CAD build for the part. Positions are in the model's coordinates, mm. Face numbers are marked on the shaded views. Coordinates: 2 decimals unless noted, no trailing zeros. Order: outer loops, then holes, each group sorted by start corner. A loop starts at its lowest first (then second) coordinate and runs counter-clockwise, first axis right, second up. Notation, with made-up numbers: M -4.75,60 L 13.25,60 A5 cw 13.25,64 Z; hole C -35.75,42.25 d3. An arc over 180 degrees is marked long. Write item = value, one per line.
from build123d import *

# Parameters (mm, degrees)
F1_R      = 645.16
F3_DEPTH  = 64.516
F2_R      = 241.935
F4_DEPTH  = 645.16
F0_R      = 65.151
F5_DEPTH  = 645.161
F6_R      = 64.516377
F7_DEPTH  = 127000
F8_R      = 32.258
F10_DEPTH = 64.516
F9_R      = 32.893
F11_DEPTH = 65.786


with BuildPart() as f3:
    # F1 (on Top) → F3 (new body)
    with BuildSketch(Plane.XY):
        Circle(F1_R)
    extrude(amount=F3_DEPTH)

    # F2 (on Top) → F4 (join)
    with BuildSketch(Plane.XY):
        Circle(F2_R)
    extrude(amount=F4_DEPTH)

    # F0 (on Top) → F5 (cut, through all)
    with BuildSketch(Plane.XY):
        Circle(F0_R)
    extrude(amount=F5_DEPTH, mode=Mode.SUBTRACT)

    # F6 (on Right) → F7 (cut, symmetric)
    with BuildSketch(Plane.YZ):
        with Locations((0, 322.58)):
            Circle(F6_R)
    extrude(amount=F7_DEPTH, both=True, mode=Mode.SUBTRACT)

    # F8 (on face) → F10 (join)
    with BuildSketch(Plane.XY.offset(645.16)):
        with Locations((0, 161.29)):
            Circle(F8_R)
    extrude(amount=F10_DEPTH)

    # F9 (on face) → F11 (cut)
    with BuildSketch(Plane.XY.offset(645.16)):
        with Locations((0, -161.29)):
            Circle(F9_R)
    extrude(amount=-F11_DEPTH, mode=Mode.SUBTRACT)


with BuildPart() as f12_1:
    # F12: copy of F3
    add(f3.part.moved(Location((1879.6, 0, 0))))


solid = f3.part
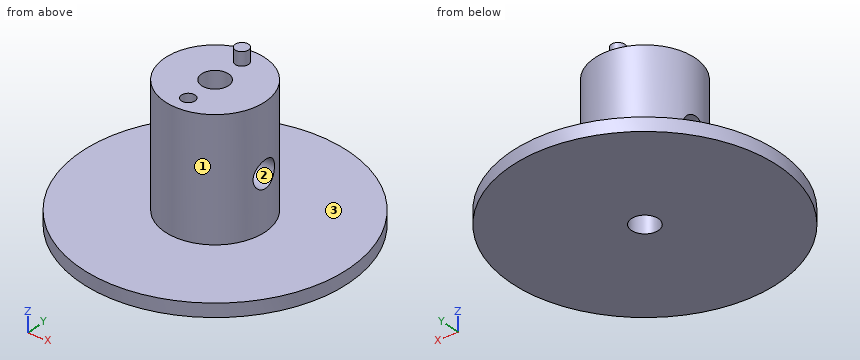
(1) Pull direction Y, two halves, no side cores. Call the marked faces 1, 2 and 3: +Y half, -Y half, draft (parallel to the pull), parting line (faces both ways), or undercut.
Evaluation:
face_1 = parting line
face_2 = undercut
face_3 = draft
(2) Slice it at B-B, the plane z = 322.58. Write the cut outline in (x, y) (3 decimals), then the cut area to 3 significant figures.
Evaluation:
outline = M -233.174,-64.516 A241.935 ccw 233.174,-64.516 L 9.071,-64.516 A65.151 cw -9.071,-64.516 Z; M -233.174,64.516 L -9.071,64.516 A65.151 cw 9.071,64.516 L 233.174,64.516 A241.935 ccw Z
area = 122,000 mm²
(3) Pin check, flat tips, straight feed: pin 1 Ø5 at (y, z) = (198, 146) entering from -X; pin 2 Ø10 at (x, y) = (-55, -18) entering from +Z. Stop position of each tip, or through.
Evaluation:
pin_1 = -142.52
pin_2 = through
(4) Wall check: line 1 (Y direction, x = 0, z = 619) (3 decimals); line 2 (X direction, y = 0, z = 484) (3 decimals); line 3 (Z direction, x = 213, y = -5). Give the ranges that are in metal, low to high. Write a range as from..to.
Evaluation:
line_1 = -241.935..-194.183, -128.397..-65.151, 65.151..241.935
line_2 = -241.935..-65.151, 65.151..241.935
line_3 = 0..258.26, 386.9..645.16
(5) Slice it at D-D, the plane y = -161.29. Write the cut outline in (x, z), then the cut area to 3 significant figures.
Evaluation:
outline = M -624.67,0 L 624.67,0 L 624.67,64.52 L 180.33,64.52 L 180.33,645.16 L 32.89,645.16 L 32.89,579.37 L -32.89,579.37 L -32.89,645.16 L -180.33,645.16 L -180.33,64.52 L -624.67,64.52 Z
area = 286,000 mm²
(6) Slice it at A-A, the plane y = 0. Write the cut outline in (x, z) (3 decimals).
Evaluation:
outline = M -645.16,0 L -65.151,0 L -65.151,258.064 L -241.935,258.064 L -241.935,64.516 L -645.16,64.516 Z; M -241.935,387.096 L -65.151,387.096 L -65.151,645.16 L -241.935,645.16 Z; M 65.151,0 L 645.16,0 L 645.16,64.516 L 241.935,64.516 L 241.935,258.064 L 65.151,258.064 Z; M 65.151,387.096 L 241.935,387.096 L 241.935,645.16 L 65.151,645.16 Z
(7) Slice it at C-C, the plane z = 404. Write the cut outline in (x, y) (3 decimals).
Evaluation:
outline = C 0,0 d483.87; hole C 0,0 d130.302
